Verification items for the finished model (mm, model axes). Face numbers are marked on the shaded views. A direction names the side the tool comes from. Coordinates: 2 decimals unless noted, no trailing zeros. Order: outer loops, then holes, each group sorted by start corner. A loop starts at its lowest first (then second) coordinate and runs counter-clockwise, first axis right, second up. Notation, with made-up numbers: (6, -27) - (38, -27) arc R22 ccw to (38, -12) - close; hole circle Ø10 at (-20, -27.75). An arc over 180 degrees is marked (long way). One line per question, with ' | ' between items. Start each with the question number.
from build123d import *

# Parameters (mm, degrees)
SKETCH1_R           = 25
BOSS_EXTRUDE1_DEPTH = 25
SKETCH2_W           = 30
SKETCH2_H           = 12.964212382
BOSS_EXTRUDE2_DEPTH = 25
FILLET1_R           = 12
FILLET2_R           = 1
FILLET3_R           = 3
SKETCH3_R           = 5
CUT_EXTRUDE1_DEPTH  = 12.964212381
FILLET4_R           = 6


with BuildPart() as part:
    # Sketch1 → Boss-Extrude1 (new body)
    with BuildSketch(Plane.XY):
        Circle(SKETCH1_R)
    extrude(amount=BOSS_EXTRUDE1_DEPTH)

    # Sketch2 → Boss-Extrude2 (add)
    with BuildSketch(Plane.XY.offset(25)):
        Rectangle(SKETCH2_W, SKETCH2_H)
    extrude(amount=BOSS_EXTRUDE2_DEPTH)

    # Fillet1
    fillet1_edges = [part.edges().sort_by_distance(p)[0] for p in [
        (15, 0, 50),
        (-15, 0, 50),
    ]]
    fillet(fillet1_edges, radius=FILLET1_R)

    # Fillet2
    fillet2_edges = [part.edges().sort_by_distance(p)[0] for p in [
        (15, 0, 25),
        (-15, 0, 25),
    ]]
    fillet(fillet2_edges, radius=FILLET2_R)

    # Fillet3
    fillet3_edges = [part.edges().sort_by_distance(p)[0] for p in [
        (0, -6.482106191, 25),
    ]]
    fillet(fillet3_edges, radius=FILLET3_R)
    fillet3_2_edges = [part.edges().sort_by_distance(p)[0] for p in [
        (0, 6.482106191, 25),
    ]]
    fillet(fillet3_2_edges, radius=FILLET3_R)

    # Sketch3 → Cut-Extrude1 (cut)
    with BuildSketch(Plane.XZ.offset(6.482106191)):
        with Locations(Location((0, 41, 0), (0, 0, 270))):
            Circle(SKETCH3_R)
    extrude(amount=-CUT_EXTRUDE1_DEPTH, mode=Mode.SUBTRACT)

    # Fillet4
    fillet4_edges = [part.edges().sort_by_distance(p)[0] for p in [
        (-25, 0, 25),
    ]]
    fillet(fillet4_edges, radius=FILLET4_R)


solid = part.part
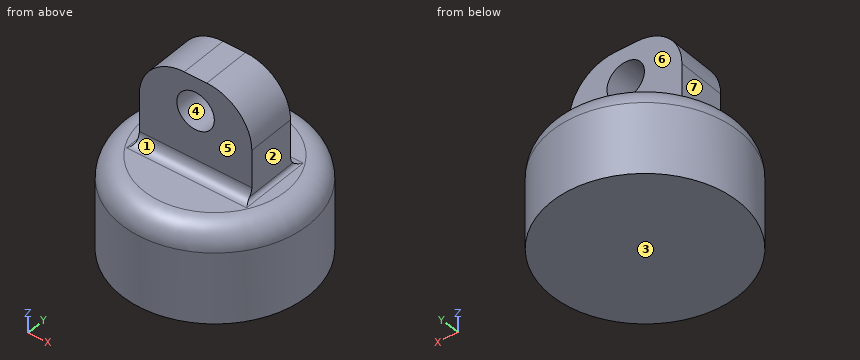
Item 1: Set-up check for the marked faces 5, 6 and 7: record each of +Z, -Z, +X, -X, +Y, -Y from which the full face is reachable in a straight line by a thin tool's end or side.
Item 2: Section check B-B (z = 41). Record the cut outline in (x, y).
Item 3: Thickness scan on probe 1 along Z at (x, y) = (1, 16); probe 2 along Y at (x, z) = (8.5, 40); probe 3 along X at (y, z) = (5.5, 40.5). Record the ranges inside material, lowest first. Write a range as from..to.
Item 4: Section check C-C (z = 13.5). Record the cut outline in (x, y), then the cut area to 3 significant figures.
Item 5: Gauge pin test, flat ends, axial feed: pin 1 (5 mm diameter, centred on y = -4.5, z = 19.5, fed in from -X); pin 2 (1.5 mm diameter, centred on x = -12, z = 14.5, fed in from +Y); pin 3 (1.5 mm diameter, centred on x = 1, y = 15.5, fed in from +Z); pin 4 (8 mm diameter, centred on x = 0, z = 41, fed in from -Y). Record the tip position at first contact, or that the pin passes through.
Item 6: Mould release check, pull along Z, two halves, no side actions. Record for the marked faces 1, 2, 3 and 4: +Z half, -Z half, draft (parallel to the pull), parting line (faces both ways), or undercut.
Item 7: Section check A-A (y = 0). Record the cut outline in (x, z), then the cut area to 3 significant figures.
Completed:
1) face 5: +Z, +X, -X, -Y | face 6: +Z, +X, -X, +Y | face 7: +Z, -X, +Y, -Y
2) outline: (-14.62, -6.48) - (-5, -6.48) - (-5, 6.48) - (-14.62, 6.48) - close; (5, -6.48) - (14.62, -6.48) - (14.62, 6.48) - (5, 6.48) - close
3) probe 1: z = 0..25 | probe 2: y = -6.48..6.48 | probe 3: x = -14.74..-4.97, 4.97..14.74
4) outline: circle Ø50 at (0, 0) | area: 1,960 mm^2
5) pin 1: stops at x = -24.92 | pin 2: stops at y = 22.33 | pin 3: stops at z = 25 | pin 4: passes through
6) face 1: +Z half | face 2: draft | face 3: -Z half | face 4: undercut
7) outline: (-25, 0) - (25, 0) - (25, 19) arc R6 ccw to (19, 25) - (16, 25) arc R1 cw to (15, 26) - (15, 38) arc R12 ccw to (3, 50) - (-3, 50) arc R12 ccw to (-15, 38) - (-15, 26) arc R1 cw to (-16, 25) - (-19, 25) arc R6 ccw to (-25, 19) - close; hole circle Ø10 at (0, 41) | area: 1,840 mm^2
